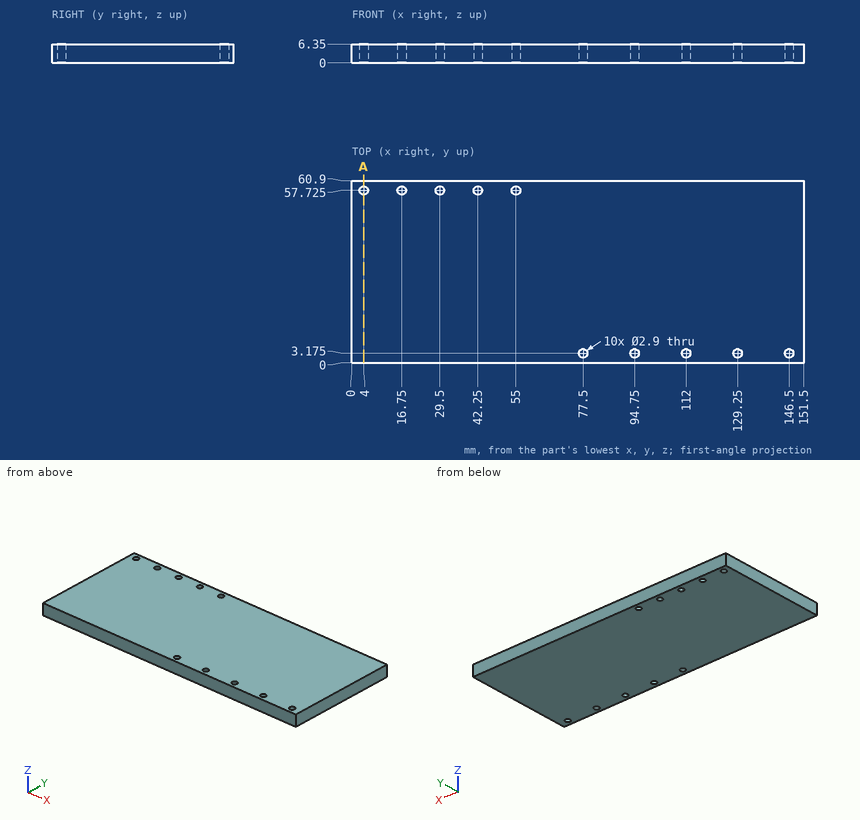
Design review of the part shown in the three views and the two pictorial views. Dimensions are in mm from the part's minimum x, y and z. Round coordinates to 2 decimals unless told otherwise and drop trailing zeros. Write each loop counter-clockwise with the first axis right and the second up, starting at its lowest first coordinate (ties: lowest second). Pieces come first, ordered by that corner, then holes.
Item 1: We need section A-A on x = 4. Write out the cut boundary in (y, z) (3 decimals), and give its area (3 significant figures).
Item 2: For probe 1 along Y at (x, z) = (42.25, 2) (3 decimals); probe 2 along X at (y, z) = (3.5, 5); probe 3 along Y at (x, z) = (112, 3.5) (3 decimals), list the stretches that pass through material, from the lowest coordinate up.
Item 3: Clearance check with flat-ended pins moving along their axes: pin 1 Ø2.5 at (x, y) = (77.5, 3.17) entering from -Z; pin 2 Ø1.5 at (y, z) = (9, 5.5) entering from -X. State where each tip first meets the part, or that it passes through.
Returned:
1. outline: (0, 0) - (56.275, 0) - (56.275, 6.35) - (0, 6.35) - close; (59.175, 0) - (60.9, 0) - (60.9, 6.35) - (59.175, 6.35) - close
1. area: 368 mm2
2. probe 1: y = 0 to 56.275, 59.175 to 60.9
2. probe 2: x = 0 to 76.09, 78.91 to 93.34, 96.16 to 110.59, 113.41 to 127.84, 130.66 to 145.09, 147.91 to 151.5
2. probe 3: y = 0 to 1.725, 4.625 to 60.9
3. pin 1: passes through
3. pin 2: stops at x = 0
